Design review of the part shown in the three views and the two pictorial views. Dimensions are in mm from the part's minimum x, y and z. Round coordinates to 2 decimals unless told otherwise and drop trailing zeros. Loops run counter-clockwise (first coordinate to the right, second up) from the corner with the lowest first, then second, coordinate; pieces in that order, holes last. Notation, with made-up numbers: (42.25, 3) - (83.25, 3) arc R17 cw to (83.25, 33) - close; hole circle Ø10 at (-25, 39.5). An arc over 180 degrees is marked (long way). Return JSON: item names as keys, results as strings. Group by question number.
(1) We need section A-A, the plane x = 10. Write out the cut boundary in (y, z).
(2) Wall thickness on L1, parallel to Z at x = 10, y = 0.2; L2, parallel to X at y = 0.2, z = 5; L3, parallel to Y at x = 18, z = 1: over which ranges is each line inside the solid? List them lowest first. Write a range as [from, to].
(3) We need section D-D, the plane x = 18.25. Write out the cut boundary in (y, z).
(4) We need section B-B, the plane z = 5. Write out the cut boundary in (x, y), and give its area (4 significant figures).
(5) The part is to be moulded in two halves that separate along X. For the marked faces 1, 2 and 3, say which applies: pulls with the +X half, pulls with the -X half, needs draft (parallel to the pull), parting line crosses it, or undercut.
(6) We need section C-C, the plane z = 9.25. Write out the cut boundary in (x, y), and give its area (3 significant figures).
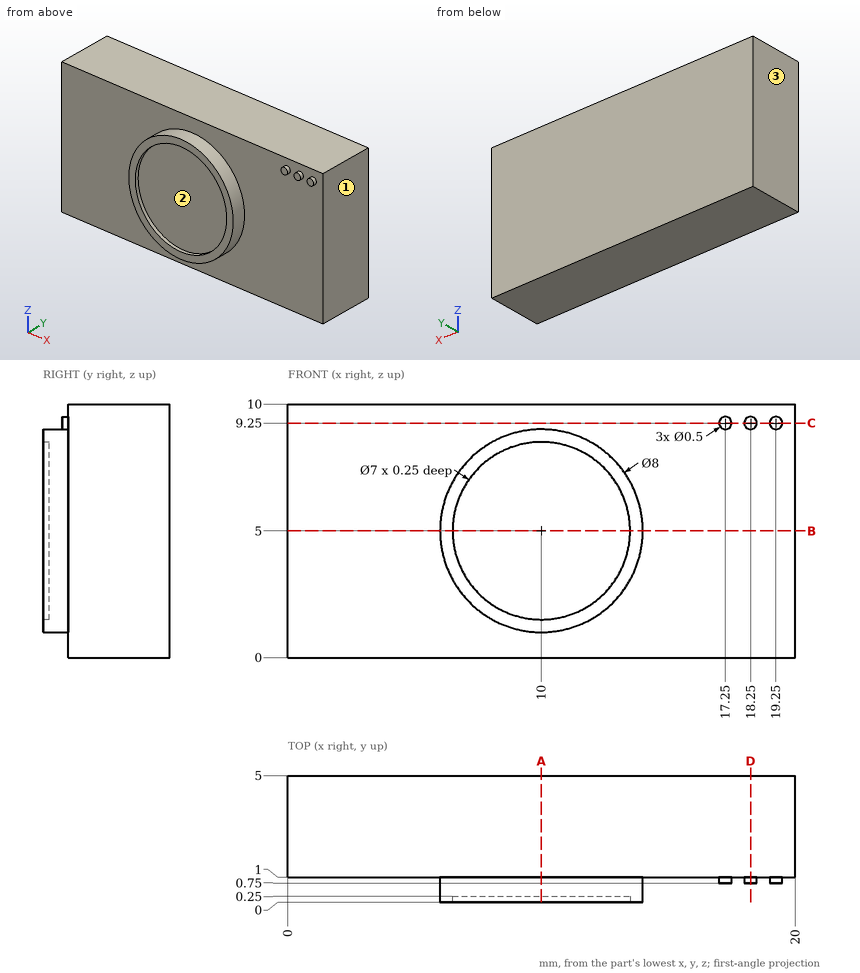
Solutions:
{
 "1": {"outline": "(0, 1) - (1, 1) - (1, 0) - (5, 0) - (5, 10) - (1, 10) - (1, 9) - (0, 9) - (0, 8.5) - (0.25, 8.5) - (0.25, 1.5) - (0, 1.5) - close"},
 "2": {"L1": "[1, 1.5], [8.5, 9]", "L2": "[6, 6.5], [13.5, 14]", "L3": "[1, 5]"},
 "3": {"outline": "(0.75, 9) - (1, 9) - (1, 0) - (5, 0) - (5, 10) - (1, 10) - (1, 9.5) - (0.75, 9.5) - close"},
 "4": {"outline": "(0, 1) - (6, 1) - (6, 0) - (6.5, 0) - (6.5, 0.25) - (13.5, 0.25) - (13.5, 0) - (14, 0) - (14, 1) - (20, 1) - (20, 5) - (0, 5) - close", "area": "86.25 mm^2"},
 "5": {"face 1": "pulls with the +X half", "face 2": "undercut", "face 3": "pulls with the -X half"},
 "6": {"outline": "(0, 1) - (17, 1) - (17, 0.75) - (17.5, 0.75) - (17.5, 1) - (18, 1) - (18, 0.75) - (18.5, 0.75) - (18.5, 1) - (19, 1) - (19, 0.75) - (19.5, 0.75) - (19.5, 1) - (20, 1) - (20, 5) - (0, 5) - close", "area": "80.4 mm^2"}
}
